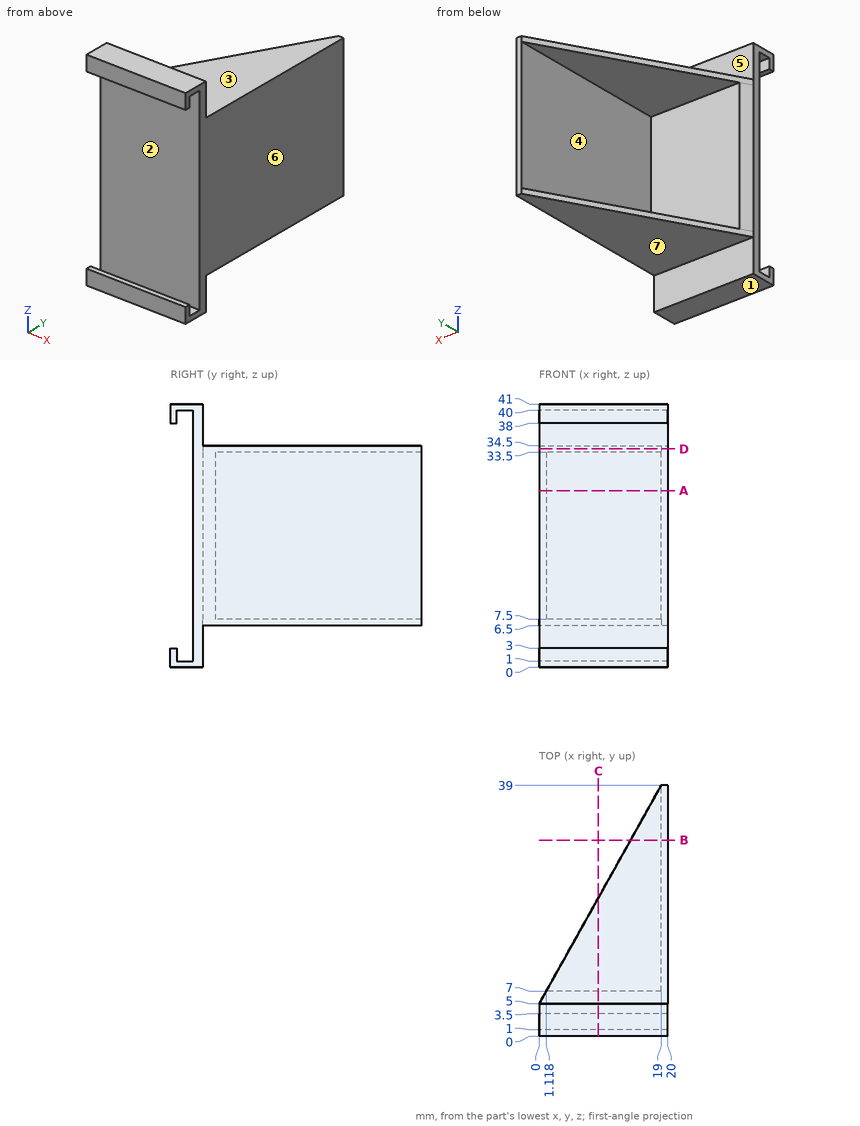
The drawing under review shows one solid part. Ordinate dimensions are in mm from its lowest x, y, z. A direction names the side the tool comes from. Give positions to 0.01 mm unless a question says otherwise; leave off trailing zeros. Loops run counter-clockwise (first coordinate to the right, second up) from the corner with the lowest first, then second, coordinate; pieces in that order, holes last. Notation, with made-up numbers: M 28.5,43 L 44.5,43 A25 ccw 44.5,61 Z; hole C 12,3.5 d4. An arc over 180 degrees is marked long. One line per item, written item: value. Start each with the question number.
Q1. Draft analysis for pull direction Z (two halves, no side actions). For the marked faces 1, 2 and 3, state which applies: released by +Z, released by -Z, zero draft, split by the parting line, or undercut.
Q2. Add section A-A (z = 27.5). Give the boundary of the cut face in (x, y).
Q3. Machinability: for the marked faces 4, 5, 6 and 7, which of the approach directions +Z, -Z, +X, -X, +Y, -Y give a long, thin tool a straight path to every point of the face, cutting with its end or side? Answer none if there is none.
Q4. Add section D-D (z = 34). Give the boundary of the cut face in (x, y), and give its area (3 significant figures).
Q5. Clearance check with flat-ended pins moving along their axes: pin 1 Ø6 at (x, z) = (13.5, 28) entering from -Y; pin 2 Ø12 at (x, y) = (15.5, 15) entering from +Z; pin 3 Ø6 at (x, z) = (6, 22) entering from +Y; pin 4 Ø1.1 at (x, y) = (12, 0.5) entering from -Z. State where each tip first meets the part, or that it passes through.
Q6. For L1, parallel to Y at x = 17.75, z = 38.5; L2, parallel to Z at x = 11, y = 22.5; L3, parallel to Z at x = 13, y = 3, list the stretches that pass through material, from the lowest coordinate up.
Q7. Add section C-C (x = 9.25). Give the boundary of the cut face in (y, z).
Q8. Add section B-B (y = 30.5). Give the boundary of the cut face in (x, z).
Reply:
1. face 1: released by -Z
1. face 2: undercut
1. face 3: released by +Z
2. outline: M 0,3.5 L 20,3.5 L 20,39 L 19,39 L 19,7 L 1.12,7 L 0,5 Z
3. face 4: -X, +Y
3. face 5: +Z, +X, -X, +Y
3. face 6: +Z, -Z, +X, +Y, -Y
3. face 7: -Z, +X, -X, +Y
4. outline: M 0,3.5 L 20,3.5 L 20,39 L 19,39 L 0,5 Z
4. area: 387 mm²
5. pin 1: y = 3.5
5. pin 2: z = 34.5
5. pin 3: y = 7
5. pin 4: z = 0
6. L1: 0 to 1, 3.5 to 5
6. L2: 6.5 to 7.5, 33.5 to 34.5
6. L3: 0 to 1, 40 to 41
7. outline: M 0,0 L 5,0 L 5,6.5 L 21.55,6.5 L 21.55,7.5 L 7,7.5 L 7,33.5 L 21.55,33.5 L 21.55,34.5 L 5,34.5 L 5,41 L 0,41 L 0,38 L 1,38 L 1,40 L 3.5,40 L 3.5,1 L 1,1 L 1,3 L 0,3 Z
8. outline: M 14.25,6.5 L 20,6.5 L 20,34.5 L 14.25,34.5 L 14.25,33.5 L 19,33.5 L 19,7.5 L 14.25,7.5 Z
